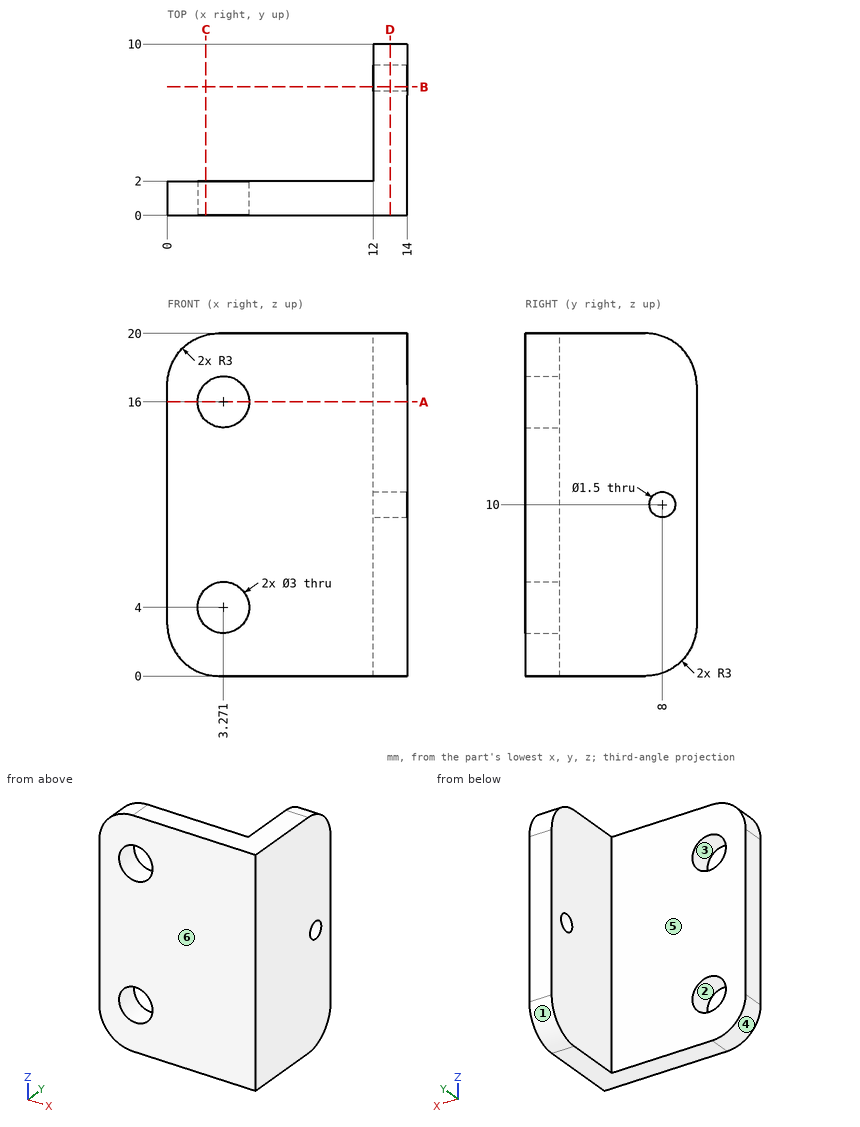
The figure shows three views and two pictorial views of one solid part (mm, origin at its lowest corner). Answer the questions. A direction names the side the tool comes from. Coordinates: 2 decimals unless noted, no trailing zeros. Loops run counter-clockwise (first coordinate to the right, second up) from the corner with the lowest first, then second, coordinate; pieces in that order, holes last. Notation, with made-up numbers: (-18, 84) -> (10, 84) arc R5 ccw to (10, 90) -> close; hole circle Ø4 at (83, 62.25). An arc over 180 degrees is marked (long way). Return JSON: item names as keys, results as strings. Group by question number.
(1) A cutting plane is placed at A-A on z = 16. Write down the section's boundary in (x, y).
(2) A cutting plane is placed at D-D on x = 13. Write down the section's boundary in (y, z), and give its area (3 significant figures).
(3) Find the intervals of material crossed by probe 1 along Y at (x, z) = (2.75, 18.5); probe 2 along X at (y, z) = (6.75, 15); probe 3 along Y at (x, z) = (12.5, 1.5), in increasing order. Write a range as from..to.
(4) Which of the six approach directions +Z, -Z, +X, -X, +Y, -Y give full straight-line access (tool end or side, diameter ignored) to the marked faces 5 and 6?
(5) Determine the mould class of the marked faces 1, 2, 3 and 4 for opening direction X: released by +X, released by -X, zero draft, split by the parting line, or undercut.
(6) A cutting plane is placed at B-B on y = 7.5. Write down the section's boundary in (x, z), and give its area (3 significant figures).
(7) A cutting plane is placed at C-C on x = 2.25. Write down the section's boundary in (y, z).
(8) Given pin 1 Ø0.9 at (y, z) = (8, 10) entering from +X; pin 2 Ø4 at (x, z) = (8.5, 15.5) entering from +Y; pin 3 Ø6 at (y, z) = (1, 15.5) entering from -X; pin 4 Ø4 at (y, z) = (4.5, 7) entering from -X, each flat-ended and moving along its own axis, determine where each tip first touches the part or whether it passes through.
The answers:
{
 "1": {"outline": "(0, 0) -> (1.77, 0) -> (1.77, 2) -> (0, 2) -> close; (4.77, 0) -> (14, 0) -> (14, 10) -> (12, 10) -> (12, 2) -> (4.77, 2) -> close"},
 "2": {"outline": "(0, 0) -> (7, 0) arc R3 ccw to (10, 3) -> (10, 17) arc R3 ccw to (7, 20) -> (0, 20) -> close; hole circle Ø1.5 at (8, 10)", "area": "194 mm^2"},
 "3": {"probe 1": "y = 0..2", "probe 2": "x = 12..14", "probe 3": "y = 0..9.6"},
 "4": {"face 5": "+Z, -Z, -X, +Y", "face 6": "+Z, -Z, +X, -X, -Y"},
 "5": {"face 1": "zero draft", "face 2": "undercut", "face 3": "undercut", "face 4": "released by -X"},
 "6": {"outline": "(12, 0.04) -> (14, 0.04) -> (14, 9.44) -> (12, 9.44) -> close; (12, 10.56) -> (14, 10.56) -> (14, 19.96) -> (12, 19.96) -> close", "area": "37.6 mm^2"},
 "7": {"outline": "(0, 0.1) -> (2, 0.1) -> (2, 2.9) -> (0, 2.9) -> close; (0, 5.1) -> (2, 5.1) -> (2, 14.9) -> (0, 14.9) -> close; (0, 17.1) -> (2, 17.1) -> (2, 19.9) -> (0, 19.9) -> close"},
 "8": {"pin 1": "passes through", "pin 2": "stops at y = 2", "pin 3": "stops at x = 0", "pin 4": "stops at x = 12"}
}
